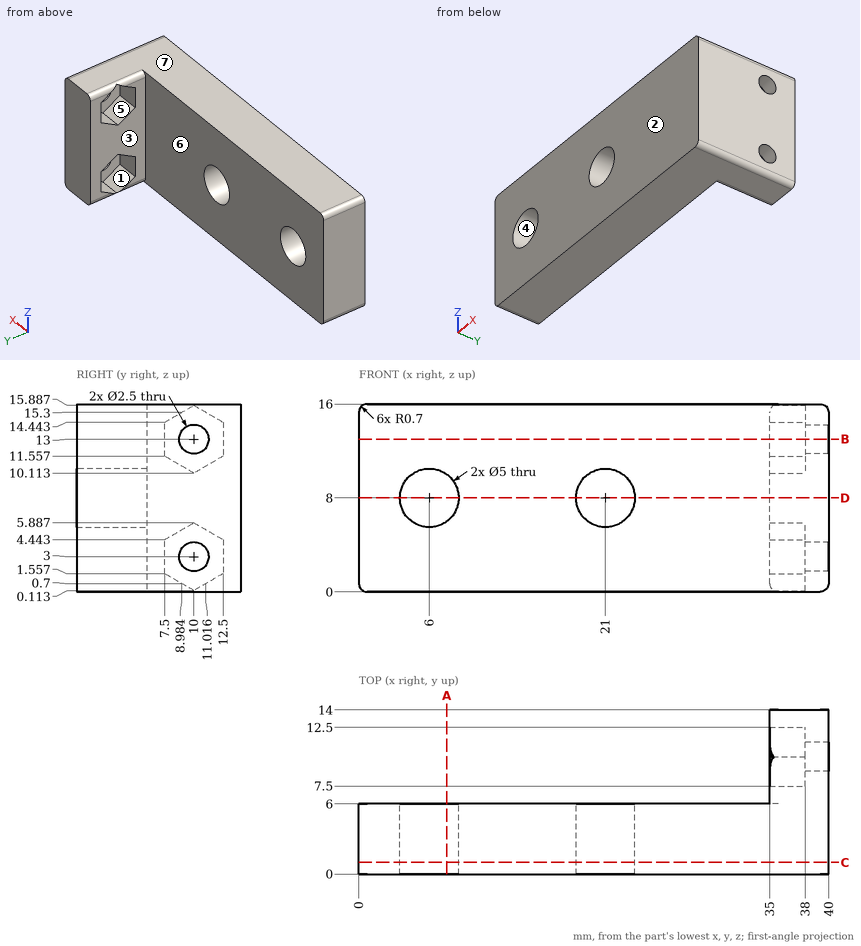
Design review of the part shown in the three views and the two pictorial views. Dimensions are in mm from the part's minimum x, y and z. A direction names the side the tool comes from. Coordinates: 2 decimals unless noted, no trailing zeros. Write each loop counter-clockwise with the first axis right and the second up, starting at its lowest first coordinate (ties: lowest second). Pieces come first, ordered by that corner, then holes.
1) We need section D-D on z = 8. State the section outline as (x, y) points, then the cut area to 3 significant figures.
2) We need section A-A on x = 7.5. State the section outline as (y, z) points.
3) The part is to be moulded in two halves that separate along Z. For the marked faces 4, 5, 6 and 7, say which applies: pulls with the +Z half, pulls with the -Z half, needs draft (parallel to the pull), parting line crosses it, or undercut.
4) To check wall thickness, follow probe 1 along X at (y, z) = (3.4, 8); probe 2 along Y at (x, z) = (38.4, 13); probe 3 along X at (y, z) = (3.5, 8.5). State the ranges of each line that lie inside material, in increasing order.
5) Clearance check with flat-ended pins moving along their axes: pin 1 Ø3 at (y, z) = (10, 13) entering from -X; pin 2 Ø5.5 at (y, z) = (9.5, 2) entering from -X; pin 3 Ø8 at (x, z) = (22, 8.5) entering from +Y. State where each tip first meets the part, or that it passes through.
6) We need section C-C on y = 1. State the section outline as (x, z) points.
7) We need section B-B on z = 13. State the section outline as (x, y) points, then the cut area to 3 significant figures.
8) Machinability: for the marked faces 1, 2 and 3, which of the approach directions +Z, -Z, +X, -X, +Y, -Y give a long, thin tool a straight path to every point of the face, cutting with its end or side? Answer none if there is none.
Answer list:
1. outline: (0, 0) - (3.5, 0) - (3.5, 6) - (0, 6) - close; (8.5, 0) - (18.5, 0) - (18.5, 6) - (8.5, 6) - close; (23.5, 0) - (40, 0) - (40, 14) - (35, 14) - (35, 6) - (23.5, 6) - close
1. area: 220 mm2
2. outline: (0, 0) - (6, 0) - (6, 6) - (0, 6) - close; (0, 10) - (6, 10) - (6, 16) - (0, 16) - close
3. face 4: undercut
3. face 5: undercut
3. face 6: needs draft
3. face 7: pulls with the +Z half
4. probe 1: x = 0 to 3.5, 8.5 to 18.5, 23.5 to 40
4. probe 2: y = 0 to 8.75, 11.25 to 14
4. probe 3: x = 0 to 3.55, 8.45 to 18.55, 23.45 to 40
5. pin 1: stops at x = 38
5. pin 2: stops at x = 35
5. pin 3: stops at y = 6
6. outline: (0, 0.7) arc R0.7 ccw to (0.7, 0) - (39.3, 0) arc R0.7 ccw to (40, 0.7) - (40, 15.3) arc R0.7 ccw to (39.3, 16) - (0.7, 16) arc R0.7 ccw to (0, 15.3) - close; hole circle Ø5 at (6, 8); hole circle Ø5 at (21, 8)
7. outline: (0, 0) - (40, 0) - (40, 8.75) - (38, 8.75) - (38, 7.5) - (35, 7.5) - (35, 6) - (0, 6) - close; (35, 12.5) - (38, 12.5) - (38, 11.25) - (40, 11.25) - (40, 14) - (35, 14) - close
7. area: 260 mm2
8. face 1: -X
8. face 2: +Z, -Z, +X, -X, -Y
8. face 3: +Z, -Z, -X, +Y
